```python
from build123d import *

# Parameters (mm, degrees)
F1_DEPTH = 10


with BuildPart() as f1:
    # F0 (on Front) → F1 (new body)
    with BuildSketch(Plane.XZ):
        with BuildLine():
            ThreePointArc((-36.543683, 48.175188), (-39.543683, 51.175188), (-42.543683, 48.175188))
            Line((-42.543683, 48.175188), (-36.543683, 48.175188))
        make_face()
        with BuildLine():
            ThreePointArc((-10.443683, 48.175188), (-19.443683, 57.175188), (-28.443683, 48.175188))
            Line((-28.443683, 48.175188), (-10.443683, 48.175188))
        make_face()
        Polygon((-36.543683, 48.175188), (-42.543683, 48.175188), (-42.543683, -61.824812), (-10.443683, -61.824812), (-10.443683, 48.175188), (-28.443683, 48.175188), align=None)
    extrude(amount=F1_DEPTH)


solid = f1.part
```
For this review, take the finished solid that the model builds, in its own axes (mm). A direction names the side the tool comes from. Round coordinates to 2 decimals unless told otherwise and drop trailing zeros. Write each loop counter-clockwise with the first axis right and the second up, starting at its lowest first coordinate (ties: lowest second). Pieces come first, ordered by that corner, then holes. Notation, with made-up numbers: (85.25, 54.25) - (94.25, 54.25) arc R31 cw to (94.25, 93.25) - close; hole circle Ø10 at (56, -38.5). An arc over 180 degrees is marked (long way). Answer as CSV lines item,"result". Start each with the question number.
(1) For pin 1 (1 mm diameter, centred on x = -37, y = -5.5, fed in from +Z), flat-tipped, find the tip position at first contact; note if it passes through.
(2) Mouldability with a two-part tool opening along X and no side actions: class faces 1 (the flat face through (-27, -5, -61.825)), 2 (the flat face through (-10.444, -5, -8)), 3 (the cylindrical face through (-39.478, -4.93, 51.174)) as +X half, -X half, draft (parallel to the pull), parting line (faces both ways), or undercut.
(3) For line 1 (Z direction, x = -34, y = -6.5); line 2 (Z direction, x = -19, y = -3.75), list the stretches that pass through material, from the lowest coordinate up.
(4) Add section A-A, the plane y = -6.5. State the section outline as (x, z) points.
(5) Add section B-B, the plane x = -29.5. State the section outline as (y, z) points, plus the area to 3 significant figures.
(6) Add section C-C, the plane x = -14. State the section outline as (y, z) points.
(7) Machinability: for faces 4 (the flat face through (-32, -5, 48.175)), 5 (the flat face through (-42.544, -5, -6)), which of the approach directions +Z, -Z, +X, -X, +Y, -Y give a long, thin tool a straight path to every point of the face, cutting with its end or side? Answer none if there is none.
From the geometry:
1,pin 1,"stops at z = 50.37"
2,face 1,"draft"
2,face 2,"+X half"
2,face 3,"undercut"
3,line 1,"z = -61.82 to 48.18"
3,line 2,"z = -61.82 to 57.16"
4,outline,"(-42.54, -61.82) - (-10.44, -61.82) - (-10.44, 48.18) arc R9 ccw to (-28.44, 48.18) - (-36.54, 48.18) arc R3 ccw to (-42.54, 48.18) - close"
5,outline,"(-10, -61.82) - (0, -61.82) - (0, 48.18) - (-10, 48.18) - close"
5,area,"1,100 mm²"
6,outline,"(-10, -61.82) - (0, -61.82) - (0, 55.34) - (-10, 55.34) - close"
7,face 4,"+Z, +Y, -Y"
7,face 5,"+Z, -Z, -X, +Y, -Y"
